from build123d import *

# Parameters (mm, degrees)
BOSS_EXTRUDE1_DEPTH      = 2.5
SKETCH2_R                = 1.2
CUT_EXTRUDE1_DEPTH       = 15.715298162
BOSS_EXTRUDE2_REACH      = 42.215
BOSS_EXTRUDE2_END_RADIUS = 7
BOSS_EXTRUDE2_START      = -25.5
SKETCH6_W                = 4
SKETCH6_H                = 5
BOSS_EXTRUDE4_DEPTH      = 1.5
FILLET1_R                = 1.5
SKETCH8_R                = 1.2
CUT_EXTRUDE3_DEPTH       = 34.395957839


with BuildPart() as part:
    # Sketch1 → Boss-Extrude1 (new, symmetric)
    with BuildSketch(Plane.XY):
        with BuildLine():
            Line((5.5, 0), (12.7, 0))
            Line((12.7, 0), (12.7, -1.5))
            Line((12.7, -1.5), (6.837397166, -1.5))
            ThreePointArc((6.837397166, -1.5), (0, -7), (-6.837397166, -1.5))
            Line((-6.837397166, -1.5), (-12.7, -1.5))
            Line((-12.7, -1.5), (-12.7, 0))
            Line((-12.7, 0), (-5.5, 0))
            ThreePointArc((-5.5, 0), (0, -5.5), (5.5, 0))
        make_face()
    extrude(amount=BOSS_EXTRUDE1_DEPTH, both=True)

    # Sketch2 → Cut-Extrude1 (cut, through all)
    with BuildSketch(Plane(origin=(0, 0, 0), x_dir=(1, 0, 0), z_dir=(0, 1, 0))):
        with Locations(Location((-10.2, 0, 0), (0, 0, 270))):
            Circle(SKETCH2_R)
        with Locations(Location((10.2, 0, 0), (0, 0, 270))):
            Circle(SKETCH2_R)
    extrude(amount=-CUT_EXTRUDE1_DEPTH, mode=Mode.SUBTRACT)

    # Boss-Extrude2: up to this cylinder (the profile starts outside it)
    boss_extrude2_end = Plane(origin=(0, 0, 0), z_dir=(0, 0, -1)) * Cylinder(BOSS_EXTRUDE2_END_RADIUS, 99.43, mode=Mode.PRIVATE)
    # Sketch6 → Boss-Extrude2 (add, up to the surface)
    with BuildSketch(Plane(origin=(0, 0, 0), x_dir=(1, 0, 0), z_dir=(0, 1, 0)).offset(BOSS_EXTRUDE2_START), mode=Mode.PRIVATE) as boss_extrude2_sk1:
        Rectangle(SKETCH6_W, SKETCH6_H)
    boss_extrude2_tool1 = extrude(boss_extrude2_sk1.sketch, amount=BOSS_EXTRUDE2_REACH, mode=Mode.PRIVATE) - boss_extrude2_end
    add(boss_extrude2_tool1.solids().sort_by_distance((0, -25.5, 0))[0])

    # Sketch7 → Boss-Extrude4 (add)
    with BuildSketch(Plane.XZ.offset(25.5)):
        Polygon((3.5, -2.5), (-3.5, -2.5), (-3.5, 2.5), (-12.7, 2.5), (-12.7, 15), (12.7, 15), (12.7, 2.5), (3.5, 2.5), align=None)
    extrude(amount=BOSS_EXTRUDE4_DEPTH)

    # Fillet1
    fillet1_edges = [part.edges().sort_by_distance(p)[0] for p in [
        (2, -25.5, 0),
        (-2, -25.5, 0),
        (-6.837397166, -1.5, 0),
        (-2, -6.708203932, 0),
        (2, -6.708203932, 0),
        (6.837397166, -1.5, 0),
        (3.5, -26.25, 2.5),
        (-3.5, -26.25, 2.5),
        (0, -25.5, 2.5),
    ]]
    fillet(fillet1_edges, radius=FILLET1_R - 0.0001)  # a hair under: the kernel refuses the full size

    # Sketch8 → Cut-Extrude3 (cut, through all)
    with BuildSketch(Plane(origin=(0, 0, 0), x_dir=(1, 0, 0), z_dir=(0, 1, 0))):
        with Locations(Location((-5, -12.5, 0), (0, 0, 270))):
            Circle(SKETCH8_R)
        with Locations(Location((5, -12.5, 0), (0, 0, 270))):
            Circle(SKETCH8_R)
    extrude(amount=-CUT_EXTRUDE3_DEPTH, mode=Mode.SUBTRACT)


solid = part.part
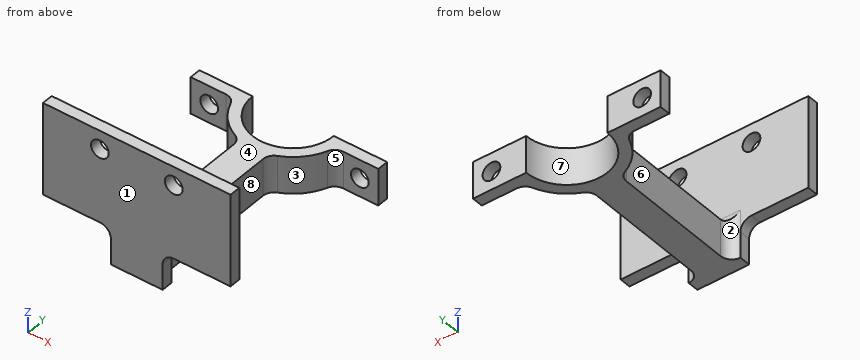
Geometry check sheet. Reference: the model listing, model coordinates, mm. Face numbers are marked on the shaded views. A direction names the side the tool comes from. Round coordinates to 2 decimals unless told otherwise and drop trailing zeros. Write each loop counter-clockwise with the first axis right and the second up, starting at its lowest first coordinate (ties: lowest second). Pieces come first, ordered by that corner, then holes. Notation, with made-up numbers: (-39.75, 10.25) -> (-6.75, 10.25) arc R22 ccw to (-6.75, 40.25) -> close; hole circle Ø5 at (-4.75, 26.5). An arc over 180 degrees is marked (long way). One line per item, written item: value. Start each with the question number.
(1) Scan lines: line 1 (X direction, y = -26.05, z = 12.5); line 2 (X direction, y = -0.3, z = 0); line 3 (Y direction, x = 10.75, z = 4). Record each from-to range of solid material in increasing order. Write a range as [from, to].
(2) Access from +Z, -Z, +X, -X, +Y, -Y to the whole of each face (thin tool, end or side, straight path). Record for the marked faces 1, 2, 3 and 4.
(3) Cross-section at D-D, the plane y = -2. Record the cut outline in (x, z).
(4) Cross-section at A-A, the plane x = -8.5. Record the cut outline in (y, z), and give its area (4 significant figures).
(5) Go/stop test with flat-tipped pins: pin 1 Ø4 at (x, z) = (10.2, 0) entering from -Y; pin 2 Ø4 at (y, z) = (-14.5, -1) entering from +X; pin 3 Ø10 at (y, z) = (-7, 4.5) entering from -X; pin 4 Ø3 at (x, z) = (-10.2, 0) entering from +Y. Record where each tip stops, or that it passes through.
(6) Draft check along Y on the marked faces 5, 6, 7 and 8. Enter one of: +Y half, -Y half, draft (parallel to the pull), parting line (faces both ways), or undercut.
(7) Cross-section at C-C, the plane z = 0. Give the number of separate pieces and of enclosed holes in the cut face, and give its area (3 significant figures).
(8) Cross-section at B-B, the plane x = 10.2. Record the cut outline in (y, z).
Answer:
1. line 1: [-12.7, -6.2], [-3.8, 3.8], [6.2, 12.7]
1. line 2: [-12.7, -11.4], [-9, -5.49], [5.49, 9], [11.4, 12.7]
1. line 3: [-27, -25.5]
2. face 1: +Z, -Z, +X, -X, -Y
2. face 2: +Z, -Z, -X
2. face 3: +Z, -Z, +X
2. face 4: +Z, +X, -X, +Y
3. outline: (-6.83, -2.5) -> (-5.12, -2.5) -> (-5.12, 2.5) -> (-6.83, 2.5) -> close; (5.12, -2.5) -> (6.83, -2.5) -> (6.83, 2.5) -> (5.12, 2.5) -> close
4. outline: (-27, 2.5) -> (-25.5, 2.5) -> (-25.5, 15) -> (-27, 15) -> close; (-1.5, -2.5) -> (0, -2.5) -> (0, 2.5) -> (-1.5, 2.5) -> close
4. area: 26.25 mm²
5. pin 1: y = -1.5
5. pin 2: x = 2
5. pin 3: x = -6.57
5. pin 4: y = 0
6. face 5: -Y half
6. face 6: undercut
6. face 7: +Y half
6. face 8: undercut
7. separate pieces: 3
7. enclosed holes: 0
7. area: 126 mm²
8. outline: (-27, 2.5) -> (-25.5, 2.5) -> (-25.5, 15) -> (-27, 15) -> close; (-1.5, -2.5) -> (0, -2.5) -> (0, -1.2) -> (-1.5, -1.2) -> close; (-1.5, 1.2) -> (0, 1.2) -> (0, 2.5) -> (-1.5, 2.5) -> close
